Part model, mm, in its own coordinate system. Face numbers are marked on the shaded views. A direction names the side the tool comes from. Give positions to 0.01 mm unless a question says otherwise; leave off trailing zeros. Write each loop counter-clockwise with the first axis right and the second up, starting at its lowest first coordinate (ties: lowest second). Pieces come first, ordered by that corner, then holes. Notation, with made-up numbers: M -17.5,9 L -6.5,9 A13 ccw -6.5,18 Z; hole C -15,14.25 d11. An arc over 180 degrees is marked long. Answer as CSV lines item,"result". Start each with the question number.
Item 1: Wall check: L1, parallel to Y at x = 5.5, z = 3.75; L2, parallel to Y at x = 0, z = -4.6; L3, parallel to Z at x = -7.25, y = 3.25. Give the ranges that are in metal, low to high. Write a range as from..to.
Item 2: Band-saw the part on A-A, the plane y = 11. List the corners of the cut face in (x, z).
Item 3: Band-saw the part on D-D, the plane z = -2. List the corners of the cut face in (x, y) (3 decimals).
Item 4: Band-saw the part on C-C, the plane x = 0. List the corners of the cut face in (y, z), then the cut area to 3 significant figures.
Item 5: Two-plate mould, pull along Y, no slides. Class the marked faces 1, 2 and 3: +Y half, -Y half, draft (parallel to the pull), parting line (faces both ways), or undercut.
Item 6: Pin check, flat tips, straight feed: pin 1 (4 mm diameter, centred on y = 5.5, z = 4, fed in from +X); pin 2 (2.5 mm diameter, centred on x = 0, z = 2, fed in from +Y). Stop position of each tip, or through.
Item 7: 3-axis set-ups, long thin cutter, end or side, ignore diameter. For the marked faces 4 and 5: which of +Z, -Z, +X, -X, +Y, -Y reach the whole face in a straight line?
Item 8: Band-saw the part on B-B, the plane x = -3.75. List the corners of the cut face in (y, z).
from build123d import *

# Parameters (mm, degrees)
SKETCH1_W           = 24
SKETCH1_H           = 10
BOSS_EXTRUDE1_DEPTH = 2
SKETCH2_W           = 24
SKETCH2_H           = 2
BOSS_EXTRUDE2_DEPTH = 16.5
SKETCH3_R           = 8
CUT_EXTRUDE1_DEPTH  = 2
CUT_EXTRUDE2_DEPTH  = 2
BOSS_EXTRUDE4_DEPTH = 1.5
BOSS_EXTRUDE5_DEPTH = 1.5


with BuildPart() as part:
    # Sketch1 → Boss-Extrude1 (new body)
    with BuildSketch(Plane(origin=(0, 0, 0), x_dir=(1, 0, 0), z_dir=(0, 1, 0))):
        Rectangle(SKETCH1_W, SKETCH1_H)
    extrude(amount=BOSS_EXTRUDE1_DEPTH)

    # Sketch2 → Boss-Extrude2 (add)
    with BuildSketch(Plane(origin=(0, 2, 0), x_dir=(1, 0, 0), z_dir=(0, 1, 0))):
        with Locations((0, 4)):
            Rectangle(SKETCH2_W, SKETCH2_H)
    extrude(amount=BOSS_EXTRUDE2_DEPTH)

    # Sketch3 → Cut-Extrude1 (cut)
    with BuildSketch(Plane.XY.offset(-3)):
        with Locations((0, 10.992781272)):
            Circle(SKETCH3_R)
    extrude(amount=-CUT_EXTRUDE1_DEPTH, mode=Mode.SUBTRACT)

    # Sketch6 → Cut-Extrude2 (cut)
    with BuildSketch(Plane.XY.offset(-3)):
        Polygon((-12, 18.5), (-8, 18.5), (-12, 14.5), align=None)
        Polygon((12, 18.5), (8, 18.5), (12, 14.5), align=None)
    extrude(amount=-CUT_EXTRUDE2_DEPTH, mode=Mode.SUBTRACT)

    # Sketch7 → Boss-Extrude4 (add)
    with BuildSketch(Plane.ZY.offset(12)):
        Polygon((-3, 2), (-3, 5), (5, 2), align=None)
    extrude(amount=-BOSS_EXTRUDE4_DEPTH)

    # Sketch8 → Boss-Extrude5 (add)
    with BuildSketch(Plane(origin=(12, 0, 0), x_dir=(0, 0, -1), z_dir=(1, 0, 0))):
        Polygon((-5, 2), (3, 2), (3, 5), align=None)
    extrude(amount=-BOSS_EXTRUDE5_DEPTH)


solid = part.part
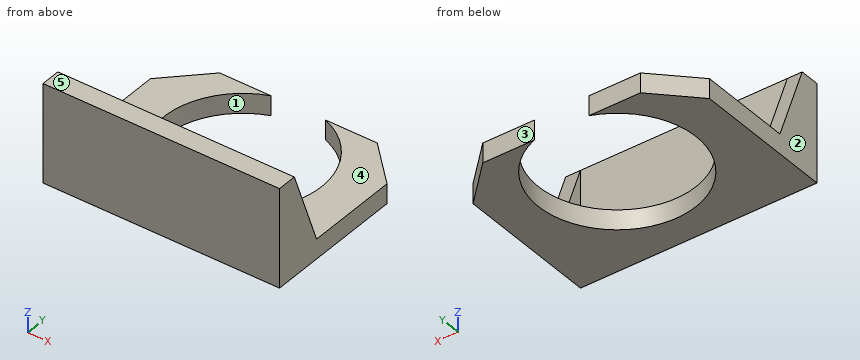
Output:
1,L1,"0..2"
1,L2,"0..2.99"
1,L3,"-5..-3"
2,outline,"M -12,-5 L -8,-5 L -8,-3 L -12,-3 Z; M 8,-5 L 12,-5 L 12,-3 L 8,-3 Z"
3,outline,"M -12,0 L 12,0 L 12,4.625 L 10.5,4.625 L 10.5,2 L -10.5,2 L -10.5,4.625 L -12,4.625 Z"
4,outline,"M 0,-5 L 2.99,-5 L 2.99,-3 L 2,-3 L 2,5 L 0,5 Z"
4,area,"22.0 mm²"
5,face 1,"undercut"
5,face 2,"draft"
5,face 3,"+Y half"
6,pin 1,"through"
6,pin 2,"y = 2"
7,face 4,"+Z, +Y"
7,face 5,"+Z, +X, -X, +Y, -Y"
8,outline,"M 0,-5 L 3.93,-5 L 3.93,-3 L 2,-3 L 2,5 L 0,5 Z; M 18.06,-5 L 18.5,-5 L 18.5,-3 L 18.06,-3 Z"
